Input: part model. Units: mm. Frame: model coordinates. Give positions to 0.01 mm unless a question says otherwise; leave off trailing zeros. Answer as a JSON object with one key per item and string values. Group by question number.
from build123d import *

# Parameters (mm, degrees)
PERFIL_COM_ALUMINIO_PERFIL_COMER_30_X_DEPTH = 300


with BuildPart() as part:
    # Esboço11 → Perfil com. aluminio PERFIL COMER. 30 X 30(1) (new body)
    with BuildSketch(Plane(origin=(0, 0, 0), x_dir=(0, 0, -1), z_dir=(1, 0, 0))):
        with BuildLine():
            Line((0, 5.872725395), (-3.872893219, 5.872725395))
            ThreePointArc((-3.872893219, 5.872725395), (-4.064234935, 5.910785628), (-4.226446609, 6.019172004))
            Line((-4.226446609, 6.019172004), (-8.073553391, 9.866278785))
            ThreePointArc((-8.073553391, 9.866278785), (-8.181939766, 10.02849046), (-8.22, 10.219832176))
            Line((-8.22, 10.219832176), (-8.22, 12.25))
            ThreePointArc((-8.22, 12.25), (-8.073553391, 12.603553391), (-7.72, 12.75))
            Line((-7.72, 12.75), (-4.5, 12.75))
            ThreePointArc((-4.5, 12.75), (-4.146446609, 12.896446609), (-4, 13.25))
            Line((-4, 13.25), (-4, 14.5))
            ThreePointArc((-4, 14.5), (-4.146446609, 14.853553391), (-4.5, 15))
            Line((-4.5, 15), (-13, 15))
            ThreePointArc((-13, 15), (-14.414213562, 14.414213562), (-15, 13))
            Line((-15, 13), (-15, 4.5))
            ThreePointArc((-15, 4.5), (-14.853553391, 4.146446609), (-14.5, 4))
            Line((-14.5, 4), (-13.25, 4))
            ThreePointArc((-13.25, 4), (-12.896446609, 4.146446609), (-12.75, 4.5))
            Line((-12.75, 4.5), (-12.75, 7.72))
            ThreePointArc((-12.75, 7.72), (-12.603553391, 8.073553391), (-12.25, 8.22))
            Line((-12.25, 8.22), (-10.219832176, 8.22))
            ThreePointArc((-10.219832176, 8.22), (-10.02849046, 8.181939766), (-9.866278785, 8.073553391))
            Line((-9.866278785, 8.073553391), (-6.019172004, 4.226446609))
            ThreePointArc((-6.019172004, 4.226446609), (-5.910785628, 4.064234935), (-5.872725395, 3.872893219))
            Line((-5.872725395, 3.872893219), (-5.872725395, 0))
            Line((-5.872725395, 0), (-5.872725395, -3.872893219))
            ThreePointArc((-5.872725395, -3.872893219), (-5.910785628, -4.064234935), (-6.019172004, -4.226446609))
            Line((-6.019172004, -4.226446609), (-9.866278785, -8.073553391))
            ThreePointArc((-9.866278785, -8.073553391), (-10.02849046, -8.181939766), (-10.219832176, -8.22))
            Line((-10.219832176, -8.22), (-12.25, -8.22))
            ThreePointArc((-12.25, -8.22), (-12.603553391, -8.073553391), (-12.75, -7.72))
            Line((-12.75, -7.72), (-12.75, -4.5))
            ThreePointArc((-12.75, -4.5), (-12.896446609, -4.146446609), (-13.25, -4))
            Line((-13.25, -4), (-14.5, -4))
            ThreePointArc((-14.5, -4), (-14.853553391, -4.146446609), (-15, -4.5))
            Line((-15, -4.5), (-15, -13))
            ThreePointArc((-15, -13), (-14.414213562, -14.414213562), (-13, -15))
            Line((-13, -15), (-4.5, -15))
            ThreePointArc((-4.5, -15), (-4.146446609, -14.853553391), (-4, -14.5))
            Line((-4, -14.5), (-4, -13.25))
            ThreePointArc((-4, -13.25), (-4.146446609, -12.896446609), (-4.5, -12.75))
            Line((-4.5, -12.75), (-7.72, -12.75))
            ThreePointArc((-7.72, -12.75), (-8.073553391, -12.603553391), (-8.22, -12.25))
            Line((-8.22, -12.25), (-8.22, -10.219832176))
            ThreePointArc((-8.22, -10.219832176), (-8.181939766, -10.02849046), (-8.073553391, -9.866278785))
            Line((-8.073553391, -9.866278785), (-4.226446609, -6.019172004))
            ThreePointArc((-4.226446609, -6.019172004), (-4.064234935, -5.910785628), (-3.872893219, -5.872725395))
            Line((-3.872893219, -5.872725395), (0, -5.872725395))
            Line((0, -5.872725395), (3.872893219, -5.872725395))
            ThreePointArc((3.872893219, -5.872725395), (4.064234935, -5.910785628), (4.226446609, -6.019172004))
            Line((4.226446609, -6.019172004), (8.073553391, -9.866278785))
            ThreePointArc((8.073553391, -9.866278785), (8.181939766, -10.02849046), (8.22, -10.219832176))
            Line((8.22, -10.219832176), (8.22, -12.25))
            ThreePointArc((8.22, -12.25), (8.073553391, -12.603553391), (7.72, -12.75))
            Line((7.72, -12.75), (4.5, -12.75))
            ThreePointArc((4.5, -12.75), (4.146446609, -12.896446609), (4, -13.25))
            Line((4, -13.25), (4, -14.5))
            ThreePointArc((4, -14.5), (4.146446609, -14.853553391), (4.5, -15))
            Line((4.5, -15), (13, -15))
            ThreePointArc((13, -15), (14.414213562, -14.414213562), (15, -13))
            Line((15, -13), (15, -4.5))
            ThreePointArc((15, -4.5), (14.853553391, -4.146446609), (14.5, -4))
            Line((14.5, -4), (13.25, -4))
            ThreePointArc((13.25, -4), (12.896446609, -4.146446609), (12.75, -4.5))
            Line((12.75, -4.5), (12.75, -7.72))
            ThreePointArc((12.75, -7.72), (12.603553391, -8.073553391), (12.25, -8.22))
            Line((12.25, -8.22), (10.219832176, -8.22))
            ThreePointArc((10.219832176, -8.22), (10.02849046, -8.181939766), (9.866278785, -8.073553391))
            Line((9.866278785, -8.073553391), (6.019172004, -4.226446609))
            ThreePointArc((6.019172004, -4.226446609), (5.910785628, -4.064234935), (5.872725395, -3.872893219))
            Line((5.872725395, -3.872893219), (5.872725395, 0))
            Line((5.872725395, 0), (5.872725395, 3.872893219))
            ThreePointArc((5.872725395, 3.872893219), (5.910785628, 4.064234935), (6.019172004, 4.226446609))
            Line((6.019172004, 4.226446609), (9.866278785, 8.073553391))
            ThreePointArc((9.866278785, 8.073553391), (10.02849046, 8.181939766), (10.219832176, 8.22))
            Line((10.219832176, 8.22), (12.25, 8.22))
            ThreePointArc((12.25, 8.22), (12.603553391, 8.073553391), (12.75, 7.72))
            Line((12.75, 7.72), (12.75, 4.5))
            ThreePointArc((12.75, 4.5), (12.896446609, 4.146446609), (13.25, 4))
            Line((13.25, 4), (14.5, 4))
            ThreePointArc((14.5, 4), (14.853553391, 4.146446609), (15, 4.5))
            Line((15, 4.5), (15, 13))
            ThreePointArc((15, 13), (14.414213562, 14.414213562), (13, 15))
            Line((13, 15), (4.5, 15))
            ThreePointArc((4.5, 15), (4.146446609, 14.853553391), (4, 14.5))
            Line((4, 14.5), (4, 13.25))
            ThreePointArc((4, 13.25), (4.146446609, 12.896446609), (4.5, 12.75))
            Line((4.5, 12.75), (7.72, 12.75))
            ThreePointArc((7.72, 12.75), (8.073553391, 12.603553391), (8.22, 12.25))
            Line((8.22, 12.25), (8.22, 10.219832176))
            ThreePointArc((8.22, 10.219832176), (8.181939766, 10.02849046), (8.073553391, 9.866278785))
            Line((8.073553391, 9.866278785), (4.226446609, 6.019172004))
            ThreePointArc((4.226446609, 6.019172004), (4.064234935, 5.910785628), (3.872893219, 5.872725395))
            Line((3.872893219, 5.872725395), (0, 5.872725395))
        make_face()
        with BuildLine():
            Line((-3.184880901, 1.488031663), (-3.963428513, 2.463089414))
            ThreePointArc((-3.963428513, 2.463089414), (-3.884059168, 3.884060272), (-2.463088278, 3.963429044))
            Line((-2.463088278, 3.963429044), (-1.488030527, 3.184881432))
            ThreePointArc((-1.488030527, 3.184881432), (-0.762142415, 3.431740597), (6.27e-07, 3.515352697))
            ThreePointArc((6.27e-07, 3.515352697), (0.762143639, 3.431740325), (1.488031663, 3.184880901))
            Line((1.488031663, 3.184880901), (2.463089414, 3.963428513))
            ThreePointArc((2.463089414, 3.963428513), (3.884060272, 3.884059168), (3.963429044, 2.463088278))
            Line((3.963429044, 2.463088278), (3.184881432, 1.488030527))
            ThreePointArc((3.184881432, 1.488030527), (3.431740597, 0.762142415), (3.515352697, -6.27e-07))
            ThreePointArc((3.515352697, -6.27e-07), (3.431740325, -0.762143639), (3.184880901, -1.488031663))
            Line((3.184880901, -1.488031663), (3.963428513, -2.463089414))
            ThreePointArc((3.963428513, -2.463089414), (3.884059168, -3.884060272), (2.463088278, -3.963429044))
            Line((2.463088278, -3.963429044), (1.488030527, -3.184881432))
            ThreePointArc((1.488030527, -3.184881432), (0.762142415, -3.431740597), (-6.27e-07, -3.515352697))
            ThreePointArc((-6.27e-07, -3.515352697), (-0.762143639, -3.431740325), (-1.488031663, -3.184880901))
            Line((-1.488031663, -3.184880901), (-2.463089414, -3.963428513))
            ThreePointArc((-2.463089414, -3.963428513), (-3.884060272, -3.884059168), (-3.963429044, -2.463088278))
            Line((-3.963429044, -2.463088278), (-3.184881432, -1.488030527))
            ThreePointArc((-3.184881432, -1.488030527), (-3.431740597, -0.762142415), (-3.515352697, 6.27e-07))
            ThreePointArc((-3.515352697, 6.27e-07), (-3.431740325, 0.762143639), (-3.184880901, 1.488031663))
        make_face(mode=Mode.SUBTRACT)
        with BuildLine():
            Line((-9.46, 13.26), (-9.46, 9.84))
            ThreePointArc((-9.46, 9.84), (-9.571299423, 9.571299423), (-9.84, 9.46))
            Line((-9.84, 9.46), (-13.26, 9.46))
            ThreePointArc((-13.26, 9.46), (-13.528700577, 9.571299423), (-13.64, 9.84))
            Line((-13.64, 9.84), (-13.64, 12.64))
            ThreePointArc((-13.64, 12.64), (-13.347106781, 13.347106781), (-12.64, 13.64))
            Line((-12.64, 13.64), (-9.84, 13.64))
            ThreePointArc((-9.84, 13.64), (-9.571299423, 13.528700577), (-9.46, 13.26))
        make_face(mode=Mode.SUBTRACT)
        with BuildLine():
            Line((13.64, 12.64), (13.64, 9.84))
            ThreePointArc((13.64, 9.84), (13.528700577, 9.571299423), (13.26, 9.46))
            Line((13.26, 9.46), (9.84, 9.46))
            ThreePointArc((9.84, 9.46), (9.571299423, 9.571299423), (9.46, 9.84))
            Line((9.46, 9.84), (9.46, 13.26))
            ThreePointArc((9.46, 13.26), (9.571299423, 13.528700577), (9.84, 13.64))
            Line((9.84, 13.64), (12.64, 13.64))
            ThreePointArc((12.64, 13.64), (13.347106781, 13.347106781), (13.64, 12.64))
        make_face(mode=Mode.SUBTRACT)
        with BuildLine():
            Line((12.64, -13.64), (9.84, -13.64))
            ThreePointArc((9.84, -13.64), (9.571299423, -13.528700577), (9.46, -13.26))
            Line((9.46, -13.26), (9.46, -9.84))
            ThreePointArc((9.46, -9.84), (9.571299423, -9.571299423), (9.84, -9.46))
            Line((9.84, -9.46), (13.26, -9.46))
            ThreePointArc((13.26, -9.46), (13.528700577, -9.571299423), (13.64, -9.84))
            Line((13.64, -9.84), (13.64, -12.64))
            ThreePointArc((13.64, -12.64), (13.347106781, -13.347106781), (12.64, -13.64))
        make_face(mode=Mode.SUBTRACT)
        with BuildLine():
            Line((-13.64, -12.64), (-13.64, -9.84))
            ThreePointArc((-13.64, -9.84), (-13.528700577, -9.571299423), (-13.26, -9.46))
            Line((-13.26, -9.46), (-9.84, -9.46))
            ThreePointArc((-9.84, -9.46), (-9.571299423, -9.571299423), (-9.46, -9.84))
            Line((-9.46, -9.84), (-9.46, -13.26))
            ThreePointArc((-9.46, -13.26), (-9.571299423, -13.528700577), (-9.84, -13.64))
            Line((-9.84, -13.64), (-12.64, -13.64))
            ThreePointArc((-12.64, -13.64), (-13.347106781, -13.347106781), (-13.64, -12.64))
        make_face(mode=Mode.SUBTRACT)
    extrude(amount=PERFIL_COM_ALUMINIO_PERFIL_COMER_30_X_DEPTH)


solid = part.part
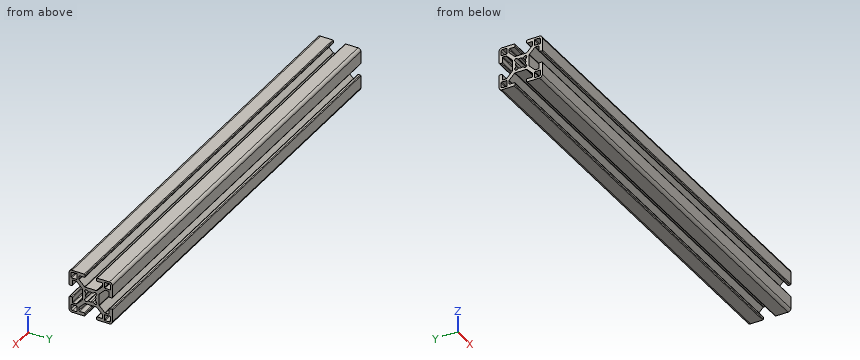
1. Section A-A (x = 282). State how many separate pieces and enclosed holes the cut face has, plus the area to 3 significant figures.
2. Contact query for flat-ended pins moving along their axis: pin 1 Ø5 at (y, z) = (0, 0.5) entering from +X; pin 2 Ø1 at (x, z) = (177.5, -14) entering from -Y; pin 3 Ø0.6 at (x, y) = (107, 13.5) entering from +Z. Output: stop coordinate, or through.
3. Line query: line 1 (Z direction, x = 216, y = 11.5); line 2 (Z direction, x = 254, y = -6.25); line 3 (Z direction, x = 117.5, y = -4.5). Output: solid intervals per line, ascending.
Working result:
{
 "1": {"separate pieces": "1", "enclosed holes": "5", "area": "317 mm^2"},
 "2": {"pin 1": "passes through", "pin 2": "stops at y = -14.94", "pin 3": "stops at z = 14.99"},
 "3": {"line 1": "z = -15 to -13.64, -9.46 to -8.22, 8.22 to 9.46, 13.64 to 15", "line 2": "z = -15 to -12.75, -8.04 to -4.46, 4.46 to 8.04, 12.75 to 15", "line 3": "z = -15 to -12.75, -6.29 to 6.29, 12.75 to 15"}
}
